Verification items for the finished model (mm, model axes). A direction names the side the tool comes from. Round coordinates to 2 decimals unless told otherwise and drop trailing zeros. Order: outer loops, then holes, each group sorted by start corner. A loop starts at its lowest first (then second) coordinate and runs counter-clockwise, first axis right, second up. Notation, with made-up numbers: (34.5, -14) -> (41.5, -14) arc R27 cw to (41.5, 25) -> close; hole circle Ø4 at (-31, 74). An arc over 180 degrees is marked (long way). Put each result on its own line as item: value.
```python
from build123d import *

# Parameters (mm, degrees)
F3_DEPTH = 4


with BuildPart() as f1:
    # F0 (on Front) → F1 (revolve)
    with BuildSketch(Plane.XZ):
        Polygon((0, 14.656888), (0, 0), (35, 0), (35, 5), (10, 5), align=None)
    revolve(axis=Axis((17.5, 0, 0), (1, 0, 0)))

    # F2 (on Right) → F3 (cut)
    with BuildSketch(Plane.YZ):
        Polygon((0, 6.928203), (-6, 3.464102), (-6, -3.464102), (0, -6.928203), (6, -3.464102), (6, 3.464102), align=None)
    extrude(amount=F3_DEPTH, mode=Mode.SUBTRACT)


solid = f1.part
```
Item 1: Depth check by flat-ended pin: pin 1 Ø5 at (x, y) = (9, 7.5) entering from +Z; pin 2 Ø2 at (x, z) = (2, 0) entering from -Y; pin 3 Ø10 at (x, z) = (16.5, -3) entering from -Y. Enter the tip coordinate at first touch or a pass-through.
Geometry check:
pin 1: z = 5.14
pin 2: y = -13.69
pin 3: y = -5
Item 2: Sectioned sample at B-B, the plane x = 14. Record the boundary of the cut face in (y, z), then the cut area to 3 significant figures.
Geometry check:
outline: circle Ø10 at (0, 0)
area: 78.5 mm2
Item 3: Release check for a two-part mould opening along Z. For faces 3 (the face through (0, 6.3, -0.2)), 4 (the face through (22.32, 4.88, -1.08)), 5 (the face through (1.972, 3.042, 5.172)) record: pulls with the +Z half, pulls with the -Z half, needs draft (parallel to the pull), parting line crosses it, or undercut.
Geometry check:
face 3: needs draft
face 4: parting line crosses it
face 5: undercut
Item 4: Tool access check on faces 1 (the face through (35, 0, 0)), 2 (the face through (2, -6, 0)). Record the directions out of +Z, -Z, +X, -X, +Y, -Y that give a thin tool (end or side, any length) a straight path to the whole face; none if there is none.
Geometry check:
face 1: +Z, -Z, +X, +Y, -Y
face 2: -X
Item 5: Material ranges on line 1 along X through (y, z) = (-5.5, -5.75); line 2 along Z through (x, y) = (33.5, 0); line 3 along Z through (x, y) = (3, 5), recorded low to high.
Geometry check:
line 1: 0 to 6.94
line 2: -5 to 5
line 3: -10.64 to -4.04, 4.04 to 10.64
Item 6: Sectioned sample at C-C, the plane x = 5. Record the boundary of the cut face in (y, z), then the cut area to 3 significant figures.
Geometry check:
outline: circle Ø19.66 at (0, 0)
area: 303 mm2
Item 7: Sectioned sample at A-A, the plane z = 0. Record the boundary of the cut face in (x, y), then the cut area to 3 significant figures.
Geometry check:
outline: (0, -14.66) -> (10, -5) -> (35, -5) -> (35, 5) -> (10, 5) -> (0, 14.66) -> (0, 6) -> (4, 6) -> (4, -6) -> (0, -6) -> close
area: 399 mm2
